from build123d import *

# Parameters (mm, degrees)
F0_W     = 457.2
F0_H     = 914.4
F1_DEPTH = 12.7
F2_W     = 457.2
F2_H     = 50.8
F3_DEPTH = 25.4
F4_R     = 19.05


with BuildPart() as f1:
    # F0 (on Top) → F1 (new body)
    with BuildSketch(Plane.XY):
        Rectangle(F0_W, F0_H)
    extrude(amount=F1_DEPTH)

    # F2 (on face) → F3 (join)
    with BuildSketch(Plane.XY.offset(12.7)):
        with Locations((0, -228.6)):
            Rectangle(F2_W, F2_H)
        with Locations((0, 228.6)):
            Rectangle(F2_W, F2_H)
    extrude(amount=F3_DEPTH)

    # F4
    f4_edges = [f1.edges().sort_by_distance(p)[0] for p in [
        (-228.6, -228.6, 38.1),
        (228.6, -228.6, 38.1),
        (228.6, 228.6, 38.1),
        (-228.6, 228.6, 38.1),
    ]]
    fillet(f4_edges, radius=F4_R)


solid = f1.part
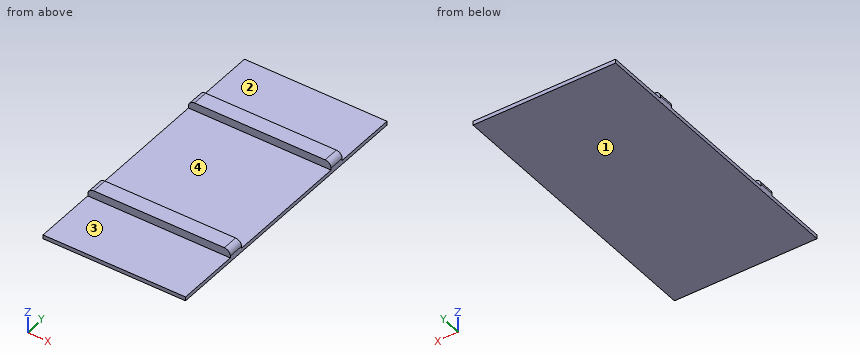
Work out the finished part from the listing and answer in its coordinate system (mm). Face numbers are marked on the shaded views. A direction names the side the tool comes from. Round coordinates to 2 decimals unless told otherwise and drop trailing zeros. Write each loop counter-clockwise with the first axis right and the second up, starting at its lowest first coordinate (ties: lowest second). Pieces come first, ordered by that corner, then holes. Notation, with made-up numbers: (14.25, 70.5) -> (54.25, 70.5) arc R31 cw to (54.25, 94.5) -> close; hole circle Ø10 at (-32, 83.5). An arc over 180 degrees is marked (long way). Write each question's results on one line, items separated by ' | '.
Item 1: Flat-ended cylindrical pins translate along their axes: P1, Ø12, axis at y = 229, z = 33.5, coming from the -X side; P2, Ø2, axis at x = -157.5, y = -325, coming from the -Z side; P3, Ø12.5, axis at x = 110.5, z = 20.5, coming from the +Y side; P4, Ø12.5, axis at x = 11, z = 28.5, coming from the -Y side. Find the tip coordinate at first contact, or state that the pin passes through.
Result set:
P1: x = -226.62 | P2: z = 0 | P3: y = 254 | P4: y = -254
Item 2: A cutting plane is placed at B-B, the plane z = 26. Determine the outline of the cut face in (x, y), plus the area to 3 significant figures.
Result set:
outline: (-227.29, -254) -> (227.29, -254) -> (227.29, -203.2) -> (-227.29, -203.2) -> close; (-227.29, 203.2) -> (227.29, 203.2) -> (227.29, 254) -> (-227.29, 254) -> close | area: 46,200 mm^2
Item 3: A cutting plane is placed at C-C, the plane y = 23.5. Determine the outline of the cut face in (x, z), plus the area to 3 significant figures.
Result set:
outline: (-228.6, 0) -> (228.6, 0) -> (228.6, 12.7) -> (-228.6, 12.7) -> close | area: 5,810 mm^2
Item 4: The mould has two halves that part along Y. Classify the marked faces 3 and 4: +Y half, -Y half, draft (parallel to the pull), parting line (faces both ways), or undercut.
Result set:
face 3: draft | face 4: undercut
Item 5: Which of the six approach directions +Z, -Z, +X, -X, +Y, -Y give full straight-line access (tool end or side, diameter ignored) to the marked faces 1 and 2?
Result set:
face 1: -Z, +X, -X, +Y, -Y | face 2: +Z, +X, -X, +Y
Item 6: A cutting plane is placed at A-A, the plane x = -155. Determine the outline of the cut face in (y, z).
Result set:
outline: (-457.2, 0) -> (457.2, 0) -> (457.2, 12.7) -> (254, 12.7) -> (254, 38.1) -> (203.2, 38.1) -> (203.2, 12.7) -> (-203.2, 12.7) -> (-203.2, 38.1) -> (-254, 38.1) -> (-254, 12.7) -> (-457.2, 12.7) -> close
Item 7: Find the intervals of material crossed by line 1 along Y through (x, z) = (-147, 24.5); line 2 along Z through (x, y) = (131, 75.5), in increasing order. Write a range as [from, to].
Result set:
line 1: [-254, -203.2], [203.2, 254] | line 2: [0, 12.7]
